Here's how the part is built. I have some questions about the finished solid (model axes, mm). A direction names the side the tool comes from. Coordinates: 2 decimals unless noted, no trailing zeros. Write each loop counter-clockwise with the first axis right and the second up, starting at its lowest first coordinate (ties: lowest second). Pieces come first, ordered by that corner, then holes. Notation, with made-up numbers: (-38.5, 60) - (-33.5, 60) arc R26 ccw to (-33.5, 82) - close; hole circle Ø6 at (-9, 9). An arc over 180 degrees is marked (long way). Answer in a Markdown table with one row per item. Add a question column.
Item 1: I'm going to push flat-ended pins straight in: pin 1 (8.5 mm diameter, centred on x = 5.08, y = 22.55, fed in from -Z); pin 2 (10 mm diameter, centred on y = 11, z = 18, fed in from +X); pin 3 (4 mm diameter, centred on y = -14.5, z = 4.5, fed in from +X); pin 4 (1.5 mm diameter, centred on y = -8, z = 14.5, fed in from +X). Where does each tip first touch, or does it pass through?
Item 2: We'd pull the mould along Y, two halves only. Please class faces 3 (the face through (-15.558, 16, 16)), 4 (the face through (27, -30.48, 13)), 5 (the face through (4.05, 17.9, 16.1)): +Y half, -Y half, draft (parallel to the pull), parting line (faces both ways), or undercut.
Item 3: Imagine slicing it at D-D (x = 17.5). Please give me the cut outline in (y, z) (3 decimals), plus the area to 3 significant figures.
Item 4: Which directions (+Z, -Z, +X, -X, +Y, -Y) give clear straight access to the entire face, cutting with the end or side of a thin tool? Please do faces 1 (the face through (15.14, 4.77, 16.1)), 2 (the face through (16, 8, 28.575)).
Item 5: If I drill on probe 1 along Y at (x, z) = (0, 11) (1 decimal); probe 2 along X at (y, z) = (19.5, 26.5); probe 3 along X at (y, z) = (-21, 4), over which ranges is the centre line in solid material (lowest first)? Write a range as from..to.
Item 6: Imagine slicing it at A-A (z = 7.5). State how many separate pieces and enclosed holes the cut face has, plus the area to 3 significant figures.
from build123d import *

# Parameters (mm, degrees)
SKETCH1_W           = 82.55
SKETCH1_H           = 76.2
BOSS_EXTRUDE1_DEPTH = 31.75
SKETCH2_R           = 4.7625
CUT_EXTRUDE1_DEPTH  = 32.75
SKETCH4_R           = 15.875
CUT_EXTRUDE3_DEPTH  = 32.75
BOSS_EXTRUDE3_DEPTH = 76.2
CUT_EXTRUDE5_DEPTH  = 77.2
CUT_EXTRUDE6_DEPTH  = 62.23
SKETCH9_W           = 31.115
SKETCH9_H           = 3.81
CUT_EXTRUDE7_DEPTH  = 25.4


with BuildPart() as part:
    # Sketch1 → Boss-Extrude1 (new body)
    with BuildSketch(Plane.XY):
        Rectangle(SKETCH1_W, SKETCH1_H)
    extrude(amount=BOSS_EXTRUDE1_DEPTH)

    # Sketch2 → Cut-Extrude1 (cut, through all)
    with BuildSketch(Plane.XY.offset(31.75)):
        with Locations((0, -23.114)):
            Circle(SKETCH2_R)
        with Locations((-5.08, 22.548849106)):
            Circle(SKETCH2_R)
        with Locations((5.08, 22.548849106)):
            Circle(SKETCH2_R)
    extrude(amount=-CUT_EXTRUDE1_DEPTH, mode=Mode.SUBTRACT)

    # Sketch4 → Cut-Extrude3 (cut, through all)
    with BuildSketch(Plane.XY.offset(31.75)):
        Circle(SKETCH4_R)
    extrude(amount=-CUT_EXTRUDE3_DEPTH, mode=Mode.SUBTRACT)

    # Sketch7 → Boss-Extrude3 (add, through all)
    with BuildSketch(Plane(origin=(0, 38.1, 0), x_dir=(1, 0, 0), z_dir=(0, 1, 0))):
        with BuildLine():
            Line((-47.639122, 0), (-41.275, 0))
            Line((-41.275, 0), (-41.275, -14.455684538))
            ThreePointArc((-41.275, -14.455684538), (-45.040781261, -7.484825392), (-47.639122, 0))
        make_face()
    boss_extrude3 = extrude(amount=-BOSS_EXTRUDE3_DEPTH)

    # Sketch6 → Cut-Extrude5 (cut, through all)
    with BuildSketch(Plane(origin=(0, 38.1, 0), x_dir=(1, 0, 0), z_dir=(0, 1, 0))):
        with BuildLine():
            Line((-41.275, -14.455684538), (-41.275, -31.75))
            Line((-41.275, -31.75), (-21.853009973, -31.75))
            ThreePointArc((-21.853009973, -31.75), (-32.727049174, -24.408972752), (-41.275, -14.455684538))
        make_face()
    cut_extrude5 = extrude(amount=-CUT_EXTRUDE5_DEPTH, mode=Mode.SUBTRACT)

    # Mirror2: Boss-Extrude3, Cut-Extrude5 across plane
    add(boss_extrude3.mirror(Plane(origin=(0, 0, 0), x_dir=(0, 0, 1), z_dir=(1, 0, 0))))
    add(cut_extrude5.mirror(Plane(origin=(0, 0, 0), x_dir=(0, 0, 1), z_dir=(1, 0, 0))), mode=Mode.SUBTRACT)


with BuildPart() as body_2:
    # Split1: the piece on the far side of the plane
    add(part.part)
    split(bisect_by=Plane(origin=(0, 31.75, 0), x_dir=(1, 0, 0), z_dir=(0, 1, 0)), keep=Keep.BOTTOM)

    # Sketch8 → Cut-Extrude6 (cut)
    with BuildSketch(Plane(origin=(0, 31.75, 0), x_dir=(1, 0, 0), z_dir=(0, 1, 0))):
        with BuildLine():
            Line((-44.689459382, -3.175), (-15.5575, -3.175))
            Line((-15.5575, -3.175), (-15.5575, -28.575))
            Line((-15.5575, -28.575), (-23.740308757, -28.575))
            ThreePointArc((-23.740308757, -28.575), (-36.495866778, -17.756285446), (-44.689459382, -3.175))
        make_face()
    cut_extrude6 = extrude(amount=-CUT_EXTRUDE6_DEPTH, mode=Mode.SUBTRACT)

    # Mirror3: Cut-Extrude6 across plane
    add(cut_extrude6.mirror(Plane(origin=(0, 0, 0), x_dir=(0, 0, 1), z_dir=(1, 0, 0))), mode=Mode.SUBTRACT)

    # Sketch9 → Cut-Extrude7 (cut)
    with BuildSketch(Plane.XY.offset(3.175)):
        with Locations((0, 29.845)):
            Rectangle(SKETCH9_W, SKETCH9_H)
    extrude(amount=CUT_EXTRUDE7_DEPTH, mode=Mode.SUBTRACT)


with BuildPart() as part_1:
    add(part.part)

    # Split1
    split(bisect_by=Plane(origin=(0, 31.75, 0), x_dir=(1, 0, 0), z_dir=(0, 1, 0)), keep=Keep.TOP)


solid = body_2.part
Here are the results:
| question | item | result |
|---|---|---|
| 1 | pin 1 | passes through |
| 1 | pin 2 | stops at x = 42.18 |
| 1 | pin 3 | stops at x = 46.92 |
| 1 | pin 4 | stops at x = 41.72 |
| 2 | face 3 | draft |
| 2 | face 4 | +Y half |
| 2 | face 5 | undercut |
| 3 | outline | (-38.1, 0) - (31.75, 0) - (31.75, 3.175) - (-30.48, 3.175) - (-30.48, 28.575) - (31.75, 28.575) - (31.75, 31.75) - (-38.1, 31.75) - close |
| 3 | area | 637 mm2 |
| 4 | face 1 | +Z, -Z |
| 4 | face 2 | +Y |
| 5 | probe 1 | y = -38.1..-27.9, -18.4..-15.9, 15.9..27.9 |
| 5 | probe 2 | x = -30.22..-27, -15.56..-8.74, -1.42..1.42, 8.74..15.56, 27..30.22 |
| 5 | probe 3 | x = -46.42..-44.39, -15.56..-4.27, 4.27..15.56, 44.39..46.42 |
| 6 | separate pieces | 2 |
| 6 | enclosed holes | 3 |
| 6 | area | 1,760 mm2 |
